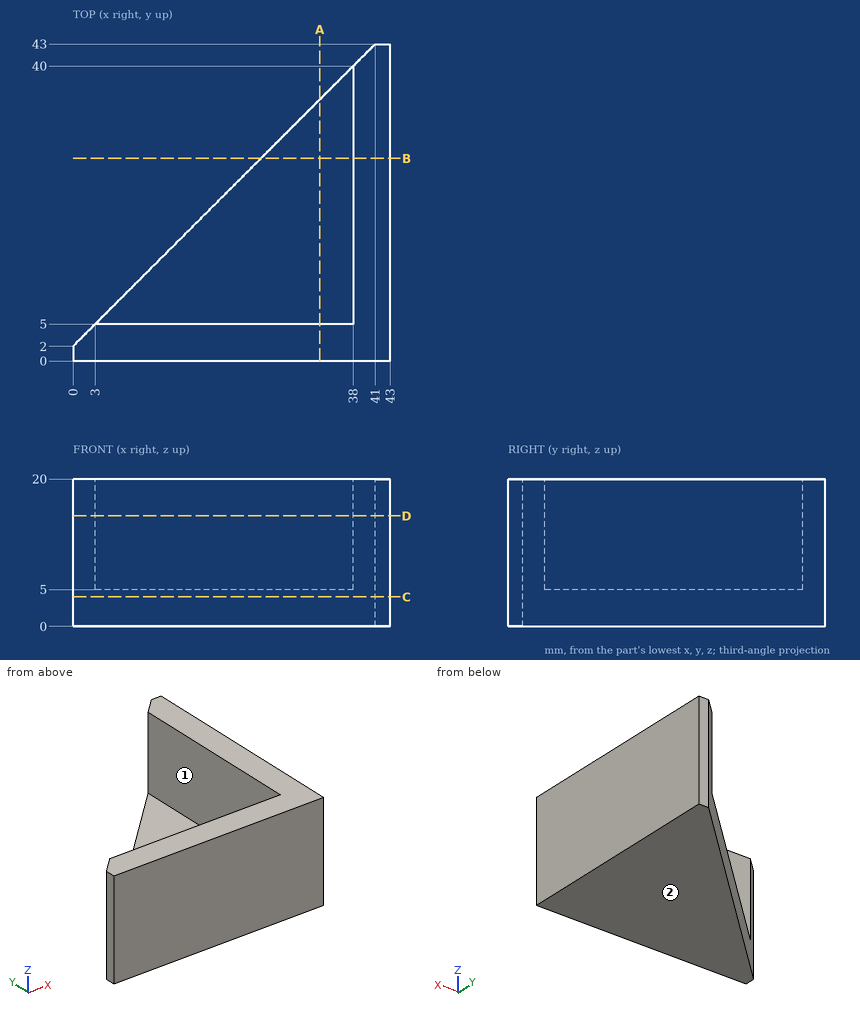
Geometry: see drawing. Coordinates: mm, zero at the bounding-box minimum. A direction names the side the tool comes from. Give positions to 0.01 mm unless a question says otherwise; leave off trailing zeros. Write each loop counter-clockwise with the first axis right and the second up, starting at its lowest first coordinate (ties: lowest second). Pieces come first, ordered by that corner, then holes. Notation, with made-up numbers: M 63.25,-29.5 L 102.25,-29.5 A25 ccw 102.25,-15.5 Z; hole C 61,87 d11. An arc over 180 degrees is marked long. Return JSON: item names as keys, results as strings. Group by question number.
1) Cut plane A-A, the plane x = 33.5. Output: boundary loops of the cut face in (y, z).
2) Cut plane B-B, the plane y = 27.5. Output: boundary loops of the cut face in (x, z).
3) Ray query, L1, parallel to X at y = 39.5, z = 17.5; L2, parallel to Z at x = 37.5, y = 25. Return the intervals inside material, ascending.
4) Cut plane D-D, the plane z = 15. Output: boundary loops of the cut face in (x, y).
5) Cut plane C-C, the plane z = 4. Output: boundary loops of the cut face in (x, y).
6) First-contact query: pin 1 Ø4.5 at (x, z) = (12, 14.5) entering from +Y; pin 2 Ø4 at (y, z) = (27.5, 6) entering from -X; pin 3 Ø10 at (x, y) = (29, 22.5) entering from +Z. Flat tips, straight axial feed; report the tip coordinate or a pass-through.
7) Set-up query: the marked faces 1 and 2. Return all of +Z, -Z, +X, -X, +Y, -Y with unobstructed straight access to the full face (end or side cutting, diameter ignored); none if empty.
Data:
{
 "1": {"outline": "M 0,0 L 35.5,0 L 35.5,5 L 5,5 L 5,20 L 0,20 Z"},
 "2": {"outline": "M 25.5,0 L 43,0 L 43,20 L 38,20 L 38,5 L 25.5,5 Z"},
 "3": {"L1": "x = 38 to 43", "L2": "z = 0 to 5"},
 "4": {"outline": "M 0,0 L 43,0 L 43,43 L 41,43 L 38,40 L 38,5 L 3,5 L 0,2 Z"},
 "5": {"outline": "M 0,0 L 43,0 L 43,43 L 41,43 L 0,2 Z"},
 "6": {"pin 1": "stops at y = 5", "pin 2": "stops at x = 23.77", "pin 3": "stops at z = 5"},
 "7": {"face 1": "+Z, -X, +Y", "face 2": "-Z, +X, -X, +Y, -Y"}
}
